Model file for the job. Use its own axes, mm. Round coordinates to 2 decimals unless told otherwise and drop trailing zeros. Loops run counter-clockwise (first coordinate to the right, second up) from the corner with the lowest first, then second, coordinate; pieces in that order, holes last. Notation, with made-up numbers: (-30.75, 87.5) - (-14.75, 87.5) arc R14 ccw to (-14.75, 112.5) - close; hole circle Ø4 at (-35, -29.5). An arc over 180 degrees is marked (long way). Use one line per item in the form item = value.
from build123d import *

# Parameters (mm, degrees)
SKETCH1_W                          = 69.85
SKETCH1_H                          = 19.05
BOSS_EXTRUDE1_DEPTH                = 1.5875
F_6_START                          = -1.5875
F_6_0_204_DIAMETER_HOLE1_OUTLINE_R = 2.5908
F_6_0_204_DIAMETER_HOLE1_DEPTH     = 3.175


# Read off the part's stored shape, not the designer's step: #6 (0.204) Diameter Hole1
with BuildPart() as part:
    # Sketch1 → Boss-Extrude1 (new, symmetric)
    with BuildSketch(Plane(origin=(0, 0, 0), x_dir=(1, 0, 0), z_dir=(0, 1, 0))):
        Rectangle(SKETCH1_W, SKETCH1_H)
    extrude(amount=BOSS_EXTRUDE1_DEPTH, both=True)

    # #6 (0.204) Diameter Hole1 outline → #6 (0.204) Diameter Hole1 (cut)
    with BuildSketch(Plane(origin=(0, 0, 0), x_dir=(1, 0, 0), z_dir=(0, 1, 0)).offset(F_6_START)):
        with Locations((-31.115, -5.715)):
            Circle(F_6_0_204_DIAMETER_HOLE1_OUTLINE_R)
        with Locations((31.115, 5.715)):
            Circle(F_6_0_204_DIAMETER_HOLE1_OUTLINE_R)
        with Locations((31.115, -5.715)):
            Circle(F_6_0_204_DIAMETER_HOLE1_OUTLINE_R)
        with Locations((-31.115, 5.715)):
            Circle(F_6_0_204_DIAMETER_HOLE1_OUTLINE_R)
    extrude(amount=F_6_0_204_DIAMETER_HOLE1_DEPTH, mode=Mode.SUBTRACT)


solid = part.part
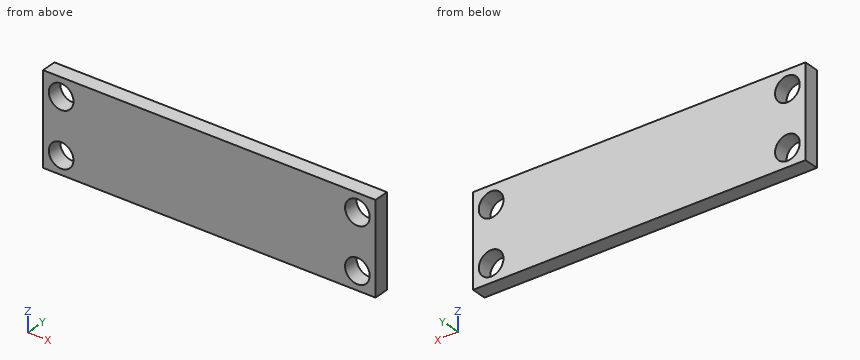
1. Flat gauge pin, fed straight in: pin 1 (4.5 mm diameter, centred on x = 31.115, z = -5.715, fed in from -Y) (3 decimals). Where does the tip first touch, or does it go through?
Geometry check:
pin_1 = through
2. Cut at C-C, the plane y = 1.05. Give the cut face in (x, z) (3 decimals), plus the area to 3 significant figures.
Geometry check:
outline = (-34.925, -9.525) - (34.925, -9.525) - (34.925, 9.525) - (-34.925, 9.525) - close; hole circle Ø5.182 at (-31.115, -5.715); hole circle Ø5.182 at (-31.115, 5.715); hole circle Ø5.182 at (31.115, -5.715); hole circle Ø5.182 at (31.115, 5.715)
area = 1,250 mm^2
3. Cut at A-A, the plane x = -31. Give the cut face in (y, z) (1 decimal).
Geometry check:
outline = (-1.6, -9.5) - (1.6, -9.5) - (1.6, -8.3) - (-1.6, -8.3) - close; (-1.6, -3.1) - (1.6, -3.1) - (1.6, 3.1) - (-1.6, 3.1) - close; (-1.6, 8.3) - (1.6, 8.3) - (1.6, 9.5) - (-1.6, 9.5) - close
4. Wall check: probe 1 along X at (y, z) = (0.2, -5.5) (3 decimals); probe 2 along X at (y, z) = (-0.25, -7) (3 decimals). Give the ranges that are in metal, low to high.
Geometry check:
probe_1 = -34.925 to -33.697, -28.533 to 28.533, 33.697 to 34.925
probe_2 = -34.925 to -33.365, -28.865 to 28.865, 33.365 to 34.925
5. Cut at B-B, the plane z = -7.5. Give the cut face in (x, y) (1 decimal), plus the area to 3 significant figures.
Geometry check:
outline = (-34.9, -1.6) - (-33, -1.6) - (-33, 1.6) - (-34.9, 1.6) - close; (-29.2, -1.6) - (29.2, -1.6) - (29.2, 1.6) - (-29.2, 1.6) - close; (33, -1.6) - (34.9, -1.6) - (34.9, 1.6) - (33, 1.6) - close
area = 198 mm^2
